```python
from build123d import *

# Parameters (mm, degrees)
ESQUISSE1_W                       = 18.518
ESQUISSE1_H                       = 32.258
BOSS_EXTRU_1_DEPTH                = 11.43
ESQUISSE2_W                       = 17.018000001
ESQUISSE2_H                       = 4.44499999
ENL_V_MAT_EXTRU_1_DEPTH           = 12.43
ESQUISSE3_W                       = 17.018000001
ESQUISSE3_H                       = 4.44499999
ENL_V_MAT_EXTRU_2_DEPTH           = 12.43
ESQUISSE4_W                       = 9.89372273
ESQUISSE4_H                       = 11.711081898
BOSS_EXTRU_2_DEPTH                = 8.5
ESQUISSE5_W                       = 2.5
ESQUISSE5_H                       = 3.438
DIAM_TRE_DU_PER_AGE_2_0_2_1_D     = 2
DIAM_TRE_DU_PER_AGE_2_0_2_1_DEPTH = 2
DIAM_TRE_DU_PER_AGE_2_0_2_2_D     = 2
DIAM_TRE_DU_PER_AGE_2_0_2_2_DEPTH = 13.438
CONG_1_R                          = 1
CONG_2_R                          = 2


with BuildPart() as part:
    # Esquisse1 → Boss.-Extru.1 (new body)
    with BuildSketch(Plane(origin=(11.43, 0, 0), x_dir=(0, 0, -1), z_dir=(1, 0, 0))):
        with Locations((7.759, 11.684)):
            Rectangle(ESQUISSE1_W, ESQUISSE1_H)
    extrude(amount=-BOSS_EXTRU_1_DEPTH)

    # Esquisse2 → Enlèv. mat.-Extru.1 (cut, through all)
    with BuildSketch(Plane.ZY):
        with Locations((-8.509, -2.222500005)):
            Rectangle(ESQUISSE2_W, ESQUISSE2_H)
    extrude(amount=-ENL_V_MAT_EXTRU_1_DEPTH, mode=Mode.SUBTRACT)

    # Esquisse3 → Enlèv. mat.-Extru.2 (cut, through all)
    with BuildSketch(Plane.ZY):
        with Locations((-8.509, 25.590500005)):
            Rectangle(ESQUISSE3_W, ESQUISSE3_H)
    extrude(amount=-ENL_V_MAT_EXTRU_2_DEPTH, mode=Mode.SUBTRACT)

    # Esquisse4 → Boss.-Extru.2 (add)
    with BuildSketch(Plane.XY.offset(1.5)):
        with Locations((5.715, 16.232232421)):
            Rectangle(ESQUISSE4_W, ESQUISSE4_H)
    extrude(amount=BOSS_EXTRU_2_DEPTH)

    # Esquisse5 → Révolution1 (revolve)
    with BuildSketch(Plane.XZ.offset(-17.399)):
        with Locations((6.965, 11.719)):
            Rectangle(ESQUISSE5_W, ESQUISSE5_H)
    revolve(axis=Axis((5.715, 17.399, 13.438), (0, 0, -1)))

    # Diamètre du perçage Ø2.0 (2)1
    with Locations(Plane.XY.offset(13.438)):
        with Locations((5.715, 17.399)):
            Hole(DIAM_TRE_DU_PER_AGE_2_0_2_1_D / 2, depth=DIAM_TRE_DU_PER_AGE_2_0_2_1_DEPTH)

    # Diamètre du perçage Ø2.0 (2)2
    with Locations(Plane(origin=(0, 0, 0), x_dir=(-1, 0, 0), z_dir=(0, 0, -1))):
        with Locations((-2.794, -1.778), (-8.636, -1.778), (-8.636, 25.146), (-2.794, 25.146)):
            Hole(DIAM_TRE_DU_PER_AGE_2_0_2_2_D / 2, depth=DIAM_TRE_DU_PER_AGE_2_0_2_2_DEPTH)

    # Congé1
    cong_1_edges = [part.edges().sort_by_distance(p)[0] for p in [
        (11.43, 27.813, 0.750000001),
        (0, 27.813, 0.750000001),
        (11.43, -4.445, 0.750000001),
        (0, -4.445, 0.750000001),
    ]]
    fillet(cong_1_edges, radius=CONG_1_R)

    # Congé2
    cong_2_edges = [part.edges().sort_by_distance(p)[0] for p in [
        (5.715, 10.376691472, 10),
        (5.715, 22.08777337, 10),
    ]]
    fillet(cong_2_edges, radius=CONG_2_R)


solid = part.part
```
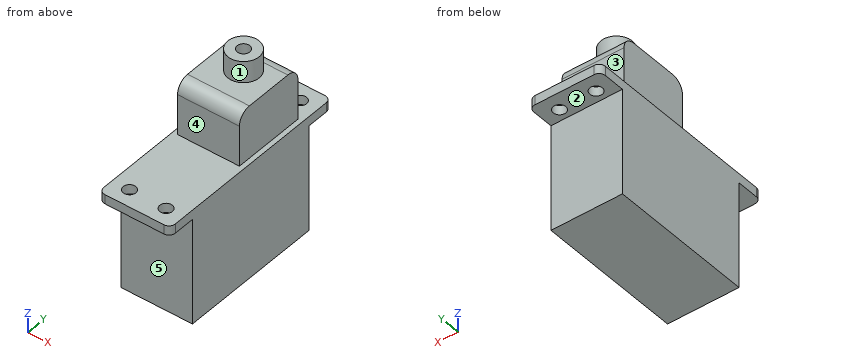
Geometry: final body of the model. Coordinates: model frame, mm. Face numbers are marked on the shaded views. A direction names the side the tool comes from. Coordinates: 2 decimals unless noted, no trailing zeros. Loops run counter-clockwise (first coordinate to the right, second up) from the corner with the lowest first, then second, coordinate; pieces in that order, holes last. Notation, with made-up numbers: (68, 6) -> (80, 6) arc R11 cw to (80, 20) -> close; hole circle Ø6 at (77.5, 38). An arc over 180 degrees is marked (long way). Use a Markdown table: item, result. Add a question column.
(1) Access query for the marked faces 1, 2, 3, 4 and 5. Directions: +Z, -Z, +X, -X, +Y, -Y. A direction counts if a zero-diameter tool reaches every point of the face in a straight line with its end or side. Return the directions, or none.
(2) Section query B-B, the plane y = 19.5. Return loops of the section in (x, z), plus the area to 3 significant figures.
(3) Line query: line 1 along Y through (x, z) = (8.25, 1) (1 decimal); line 2 along Z through (x, y) = (2, 4); line 3 along Z through (x, y) = (1.75, 16.5). Output: solid intervals per line, ascending.
(4) Section query D-D, the plane y = 23. Return loops of the section in (x, z).
(5) Section query A-A, the plane x = 2.75. Return loops of the section in (y, z) (3 decimals).
(6) Section query C-C, the plane z = -6. Return loops of the section in (x, y), plus the area to 3 significant figures.
(7) Pin query (flat end, axial travel): pin 1 Ø4 at (x, z) = (6, -10) entering from -Y; pin 2 Ø3 at (x, y) = (7, -0.5) entering from +Z; pin 3 Ø1.5 at (y, z) = (-0.5, -13) entering from +X; pin 4 Ø2.5 at (x, y) = (2.794, 25.146) entering from -Z. Return the tip coordinate at first contact, or that it passes through.
Answer:
| question | item | result |
|---|---|---|
| 1 | face 1 | +Z |
| 1 | face 2 | -Z, +X, -X, +Y |
| 1 | face 3 | +Z, +X, -X, +Y |
| 1 | face 4 | +Z, +X, -X, -Y |
| 1 | face 5 | -Z, +X, -X, -Y |
| 2 | outline | (0, -17.02) -> (11.43, -17.02) -> (11.43, 1.5) -> (10.66, 1.5) -> (10.66, 10) -> (7.07, 10) -> (7.07, 13.44) -> (4.36, 13.44) -> (4.36, 10) -> (0.77, 10) -> (0.77, 1.5) -> (0, 1.5) -> close |
| 2 | area | 305 mm^2 |
| 3 | line 1 | y = -4.4 to -2.7, -0.9 to 24.2, 26.1 to 27.8 |
| 3 | line 2 | z = -17.02 to 1.5 |
| 3 | line 3 | z = -17.02 to 10 |
| 4 | outline | (0, -17.02) -> (11.43, -17.02) -> (11.43, 1.5) -> (0, 1.5) -> close |
| 5 | outline | (-4.445, 0) -> (-2.777, 0) -> (-2.777, 1.5) -> (-4.445, 1.5) -> close; (-0.779, 0) -> (0, 0) -> (0, -17.018) -> (23.368, -17.018) -> (23.368, 0) -> (24.147, 0) -> (24.147, 1.5) -> (22.088, 1.5) -> (22.088, 8) arc R2 ccw to (20.088, 10) -> (12.377, 10) arc R2 ccw to (10.377, 8) -> (10.377, 1.5) -> (-0.779, 1.5) -> close; (26.145, 0) -> (27.813, 0) -> (27.813, 1.5) -> (26.145, 1.5) -> close |
| 6 | outline | (0, 0) -> (11.43, 0) -> (11.43, 23.37) -> (0, 23.37) -> close |
| 6 | area | 267 mm^2 |
| 7 | pin 1 | stops at y = 0 |
| 7 | pin 2 | stops at z = 1.5 |
| 7 | pin 3 | stops at x = 11.43 |
| 7 | pin 4 | stops at z = 0 |
